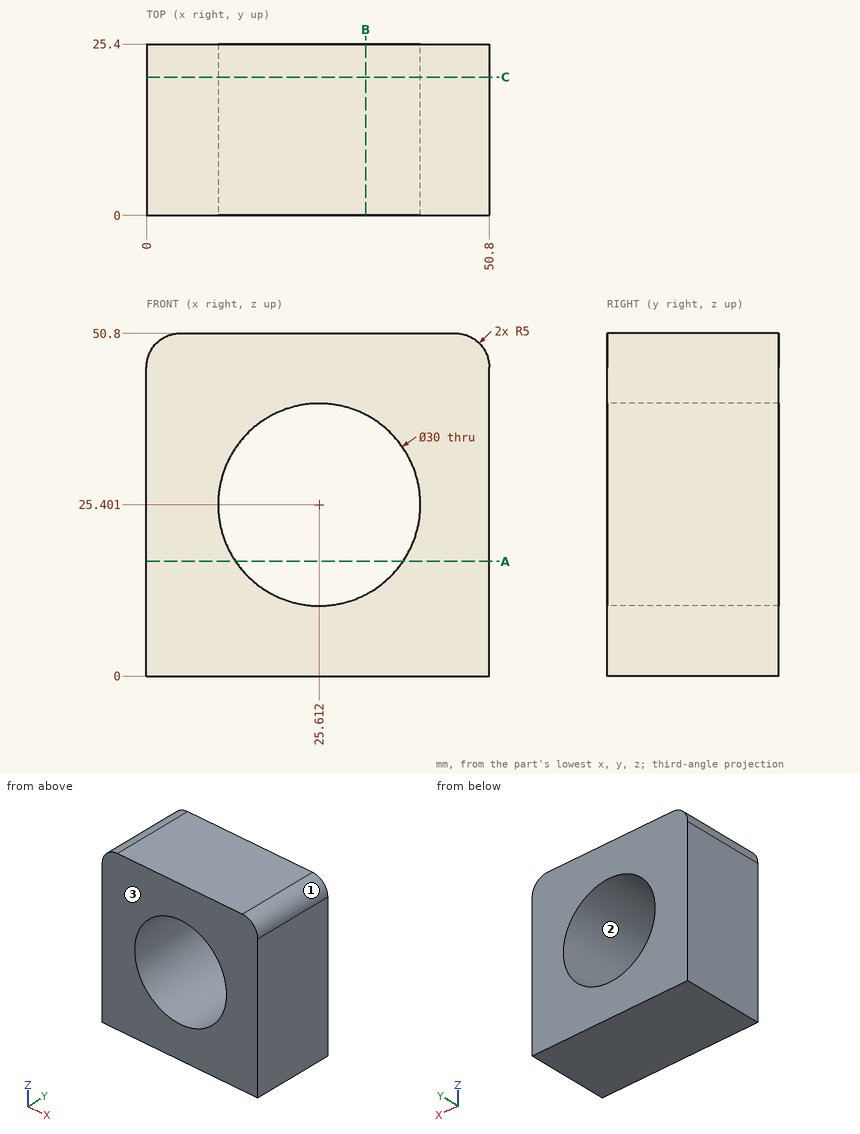
The figure shows three views and two pictorial views of one solid part (mm, origin at its lowest corner). Answer the questions. Round coordinates to 2 decimals unless told otherwise and drop trailing zeros. Order: outer loops, then holes, each group sorted by start corner. A loop starts at its lowest first (then second) coordinate and runs counter-clockwise, first axis right, second up. Notation, with made-up numbers: M 2,40 L 51,40 A27 ccw 51,67 Z; hole C 55.25,62 d5. An arc over 180 degrees is marked long. Answer in a Markdown table with one row per item. Add a question column.
1) Determine the mould class of the marked faces 1, 2 and 3 for opening direction Z: pulls with the +Z half, pulls with the -Z half, needs draft (parallel to the pull), parting line crosses it, or undercut.
2) The part is cut by section A-A on z = 17. Determine the outline of the cut face in (x, y) (1 decimal).
3) Consider line 1 along X through (y, z) = (13.5, 23) (1 decimal); line 2 along Z through (x, y) = (13, 10.25); line 3 along X through (y, z) = (8.75, 29). Determine where each line is inside the solid, lowest interval first. Write a range as from..to.
4) The part is cut by section B-B on x = 32.5. Determine the outline of the cut face in (y, z).
5) The part is cut by section C-C on y = 20.5. Determine the outline of the cut face in (x, z), plus the area to 3 significant figures.
6) A flat-ended cylindrical pin translates along its axis: pin 1 Ø24 at (x, z) = (25.61, 25.4) entering from -Y. Find the tip coordinate at first contact, or state that the pin passes through.
Findings below:
| question | item | result |
|---|---|---|
| 1 | face 1 | pulls with the +Z half |
| 1 | face 2 | undercut |
| 1 | face 3 | needs draft |
| 2 | outline | M 0,0 L 13.2,0 L 13.2,25.4 L 0,25.4 Z; M 38,0 L 50.8,0 L 50.8,25.4 L 38,25.4 Z |
| 3 | line 1 | x = 0..10.8, 40.4..50.8 |
| 3 | line 2 | z = 0..17.28, 33.52..50.8 |
| 3 | line 3 | x = 0..11.05, 40.17..50.8 |
| 4 | outline | M 0,0 L 25.4,0 L 25.4,12.08 L 0,12.08 Z; M 0,38.73 L 25.4,38.73 L 25.4,50.8 L 0,50.8 Z |
| 5 | outline | M 0,0 L 50.8,0 L 50.8,45.8 A5 ccw 45.8,50.8 L 5,50.8 A5 ccw 0,45.8 Z; hole C 25.61,25.4 d30 |
| 5 | area | 1,860 mm² |
| 6 | pin 1 | passes through |
